The model under review builds one solid part; all positions refer to its coordinate system, in mm. A direction names the side the tool comes from. Give positions to 0.01 mm unless a question says otherwise; leave off trailing zeros. Order: outer loops, then holes, each group sorted by start corner. A loop starts at its lowest first (then second) coordinate and runs counter-clockwise, first axis right, second up.
```python
from build123d import *

# Parameters (mm, degrees)
BASE_SHAPE_DEPTH            = 2
SCREW_HOLE_SKETCH_R         = 1.25
SCREW_HOLE_DEPTH            = 51.413108579
PCB_CUTOUT_SKETCH_W         = 9
PCB_CUTOUT_SKETCH_H         = 11
CAMERA_PCB_CUTOUT_DEPTH     = 1.5
CAMERA_RIBBON_ROUTING_DEPTH = 9


with BuildPart() as part:
    # Base Shape Sketch → Base Shape (new body)
    with BuildSketch(Plane(origin=(0, 0, 0), x_dir=(1, 0, 0), z_dir=(0, 1, 0))):
        with BuildLine():
            Line((0, 15.19), (38.325, 15.19))
            Line((38.325, 15.19), (38.325, 17.5294293))
            Line((38.325, 17.5294293), (47.225, 17.5294293))
            Line((47.225, 17.5294293), (47.225, -17.5294293))
            Line((47.225, -17.5294293), (36.825, -17.5294293))
            Line((36.825, -17.5294293), (36.825, -15.19))
            Line((36.825, -15.19), (0, -15.19))
            ThreePointArc((0, -15.19), (-15.19, 0), (0, 15.19))
        make_face()
    extrude(amount=BASE_SHAPE_DEPTH)

    # Screw Hole Sketch → Screw Hole (cut, through all)
    with BuildSketch(Plane(origin=(0, 2, 0), x_dir=(1, 0, 0), z_dir=(0, 1, 0))):
        with Locations(Location((8.5, 0, 0), (0, 0, 270))):
            Circle(SCREW_HOLE_SKETCH_R)
    extrude(amount=-SCREW_HOLE_DEPTH, mode=Mode.SUBTRACT)

    # Countersink Sketch → Screw Hole Countersink (revolve, cut)
    with BuildSketch(Plane.XY, mode=Mode.PRIVATE) as screw_hole_countersink_sk:
        Polygon((8.5, 2), (8.5, 0.8), (9.5, 0.8), (9.5, 1.1), (10.4, 2), align=None)
    revolve(screw_hole_countersink_sk.sketch.rotate(Axis((8.5, 2, 0), (0, -1, 0)), 90), axis=Axis((8.5, 2, 0), (0, -1, 0)), mode=Mode.SUBTRACT)

    # PCB Cutout Sketch → Camera PCB Cutout (cut)
    with BuildSketch(Plane.XZ):
        with Locations((0, -1)):
            Rectangle(PCB_CUTOUT_SKETCH_W, PCB_CUTOUT_SKETCH_H)
    extrude(amount=-CAMERA_PCB_CUTOUT_DEPTH, mode=Mode.SUBTRACT)

    # Ribbon Routing Sketch → Camera Ribbon Routing (cut)
    with BuildSketch(Plane.ZY.offset(-4.5)):
        Polygon((-6.5, 1.5), (-12.098076211, 0), (-6.5, 0), align=None)
    extrude(amount=CAMERA_RIBBON_ROUTING_DEPTH, mode=Mode.SUBTRACT)


solid = part.part
```
Item 1: Take a section at C-C (y = 0.6). Give the boundary of the cut face in (x, z) (3 decimals).
Values found:
outline: (0, -15.19) - (38.325, -15.19) - (38.325, -17.529) - (47.225, -17.529) - (47.225, 17.529) - (36.825, 17.529) - (36.825, 15.19) - (0, 15.19) arc R15.19 ccw to start; hole (-4.5, -9.859) - (4.5, -9.859) - (4.5, 4.5) - (-4.5, 4.5) - close; hole circle Ø2.5 at (8.5, 0)
Item 2: For faces 5 (the flat face through (42, 1, 17.529)), 6 (the flat face through (-4.5, 1, -2)), 7 (the flat face through (19, 1, 15.19)), 8 (the cylindrical face through (9.74, 0.68, -0.16)), 9 (the flat face through (38.325, 1, -16)), list the 3-axis set-ups (+Z, -Z, +X, -X, +Y, -Y) from which the entire face can be reached by the end or side of a thin tool; tool diameter is ignored.
Values found:
face 5: +Z, +X, -X, +Y, -Y
face 6: -Y
face 7: +Z, -X, +Y, -Y
face 8: +Y, -Y
face 9: -Z, -X, +Y, -Y
Item 3: Take a section at B-B (z = 0). Give the boundary of the cut face in (x, y) (3 decimals), and give its area (3 significant figures).
Values found:
outline: (-15.19, 0) - (-4.5, 0) - (-4.5, 1.5) - (4.5, 1.5) - (4.5, 0) - (7.25, 0) - (7.25, 1.35) - (6.6, 2) - (-15.19, 2) - close; (9.75, 0) - (47.225, 0) - (47.225, 2) - (10.4, 2) - (9.75, 1.35) - close
area: 106 mm2
Item 4: Clearance check with flat-ended pins moving along their axes: pin 1 Ø1 at (x, y) = (-0.5, 1) entering from -Z; pin 2 Ø0.8 at (y, z) = (0.5, -3.5) entering from -X; pin 3 Ø0.6 at (y, z) = (0.5, 16) entering from -X (3 decimals). State where each tip first meets the part, or that it passes through.
Values found:
pin 1: stops at z = -15.19
pin 2: stops at x = -14.87
pin 3: stops at x = 36.825
Item 5: Draft analysis for pull direction X (two halves, no side actions). For faces 1 (the flat face through (36.825, 1, 16)), 2 (the flat face through (47.225, 1, 0)), 3 (the flat face through (0, 1, 4.5)), 4 (the flat face through (23, 0, 0)), state which applies: released by +X, released by -X, zero draft, split by the parting line, or undercut.
Values found:
face 1: released by -X
face 2: released by +X
face 3: undercut
face 4: zero draft
Item 6: Take a section at A-A (x = 8.5). Give the boundary of the cut face in (y, z), and give its area (3 significant figures).
Values found:
outline: (0, -15.19) - (2, -15.19) - (2, -1.9) - (1.35, -1.25) - (0, -1.25) - close; (0, 1.25) - (1.35, 1.25) - (2, 1.9) - (2, 15.19) - (0, 15.19) - close
area: 55.3 mm2
Item 7: Take a section at D-D (z = -9). Give the boundary of the cut face in (x, y) (3 decimals), and give its area (3 significant figures).
Values found:
outline: (-12.237, 0) - (-4.5, 0) - (-4.5, 0.83) - (4.5, 0.83) - (4.5, 0) - (47.225, 0) - (47.225, 2) - (-12.237, 2) - close
area: 111 mm2
Item 8: For line 1 (X direction, y = 0.35, z = 0) (3 decimals); line 2 (Z direction, x = 24, y = 0.4); line 3 (X direction, y = 1.1, z = -2.5) (3 decimals), list the stretches that pass through material, from the lowest coordinate up.
Values found:
line 1: x = -15.19 to -4.5, 4.5 to 7.25, 9.75 to 47.225
line 2: z = -15.19 to 15.19
line 3: x = -14.983 to -4.5, 4.5 to 47.225
